Autodesk Inventor part; units mm, degrees
ref_plane "YZ Plane" through (0, 0, 0) normal (1, 0, 0) x (0, 1, 0)
ref_plane "XZ Plane" through (0, 0, 0) normal (0, 1, 0) x (-1, 0, 0)
ref_plane "XY Plane" through (0, 0, 0) normal (0, 0, 1) x (1, 0, 0)
sketch "Sketch1" plane through (0, 0, 0) normal (0, 1, 0) x (-1, 0, 0)
  line L0 (-9.9441, 7.0739) -> (9.9441, 7.0739)
  line L1 (9.9441, 7.0739) -> (9.9441, -7.0739)
  line L2 (9.9441, -7.0739) -> (-9.9441, -7.0739)
  line L3 (-9.9441, -7.0739) -> (-9.9441, 7.0739)
  line L4 (-9.9441, 7.0739) -> (9.9441, -7.0739) construction
  line L5 (9.9441, 7.0739) -> (-9.9441, -7.0739) construction
  line L6 (5.2211, 0) -> (2.6105, -4.5216)
  line L7 (2.6105, -4.5216) -> (-2.6105, -4.5216)
  line L8 (-2.6105, -4.5216) -> (-5.2211, 0)
  line L9 (-5.2211, 0) -> (-2.6105, 4.5216)
  line L10 (-2.6105, 4.5216) -> (2.6105, 4.5216)
  line L11 (2.6105, 4.5216) -> (5.2211, 0)
  point P0 (0, 0)
  point P1 (0, 0)
  dimension "d0" = 19.8882
  dimension "d1" = 14.1478
extrude "Extrusion1" add sketch "Sketch1" along normal blind 3.9688 contours L6 L7 L8 L9 L10 L11
properties part number "Wheel side stand nut"
Here's how the part is built. I have some questions about the finished solid (model axes, mm). Give positions to 0.01 mm unless a question says otherwise; leave off trailing zeros. Order: outer loops, then holes, each group sorted by start corner. A loop starts at its lowest first (then second) coordinate and runs counter-clockwise, first axis right, second up. Notation, with made-up numbers: M -17,20.5 L -2,20.5 A21 ccw -2,54.5 Z; hole C 82,8 d9. An arc over 180 degrees is marked long. Answer as a JSON object with one key per item and string values. Group by question number.
1) I'm going to push a flat-ended pin straight in: pin 1 Ø1 at (y, z) = (1.5, -1) entering from +X. Where does the tip first touch, or does it pass through?
2) Suppose I cut it at B-B, the plane x = 3.75. Write out the boundary of the cut face in (y, z).
3) Suppose I cut it at A-A, the plane y = 2.25. Write out the boundary of the cut face in (x, z), plus the area to 3 significant figures.
4) Please list where these lines run through material, in increasing order: L1, parallel to Z at x = 4.25, y = 2.2; L2, parallel to X at y = 3.8, z = -4; L3, parallel to X at y = 2, z = 3.75. Write a range as [from, to].
5) Suppose I cut it at C-C, the plane z = -2.75. Write out the boundary of the cut face in (x, y), plus the area to 3 significant figures.
6) We'd pull the mould along Y, two halves only. Please class faces 1 (the flat face through (0, 2, 4.522)), 2 (the flat face through (0, 0, 0)), 3 (the flat face through (0, 3.969, 0)): pulls with the +Y half, pulls with the -Y half, needs draft (parallel to the pull), parting line crosses it, or undercut.
Results found:
{
 "1": {"pin 1": "x = 4.93"},
 "2": {"outline": "M 0,-2.55 L 3.97,-2.55 L 3.97,2.55 L 0,2.55 Z"},
 "3": {"outline": "M -5.22,0 L -2.61,-4.52 L 2.61,-4.52 L 5.22,0 L 2.61,4.52 L -2.61,4.52 Z", "area": "70.8 mm²"},
 "4": {"L1": "[-1.68, 1.68]", "L2": "[-2.91, 2.91]", "L3": "[-3.06, 3.06]"},
 "5": {"outline": "M -3.63,0 L 3.63,0 L 3.63,3.97 L -3.63,3.97 Z", "area": "28.8 mm²"},
 "6": {"face 1": "needs draft", "face 2": "pulls with the -Y half", "face 3": "pulls with the +Y half"}
}
